For this review, take the finished solid that the model builds, in its own axes (mm). Round coordinates to 2 decimals unless told otherwise and drop trailing zeros. Order: outer loops, then holes, each group sorted by start corner. A loop starts at its lowest first (then second) coordinate and runs counter-clockwise, first axis right, second up. Notation, with made-up numbers: (-29.75, 57.25) -> (17.25, 57.25) arc R26 ccw to (17.25, 80.25) -> close; hole circle Ø5 at (-20, 45). An arc over 180 degrees is marked (long way). Answer in a Markdown table with one row per item.
```python
from build123d import *

# Parameters (mm, degrees)
SKETCH1_R               = 2
BOSS_EXTRUDE1_DEPTH     = 4
BOSS_EXTRUDE2_DEPTH     = 6
CUT_EXTRUDE1_START      = -2
CUT_EXTRUDE1_DEPTH      = 18
SKETCH4_W               = 12.2
SKETCH4_H               = 11
CUT_EXTRUDE2_DEPTH      = 10
SKETCH5_W               = 20
SKETCH5_H               = 2
BOSS_EXTRUDE3_DEPTH     = 35
CUT_EXTRUDE4_START      = -0.7
CUT_EXTRUDE4_DEPTH      = 0.7
CUT_EXTRUDE5_DEPTH      = 1
CUT_EXTRUDE6_REACH      = 144.046
SKETCH12_W              = 87
SKETCH12_H              = 2
FILLET1_R               = 10
CUT_EXTRUDE7_DEPTH      = 112.736296699
SKETCH14_W              = 20
SKETCH14_H              = 2
CUT_EXTRUDE8_DEPTH      = 142.58036587
FILLET2_R               = 10
CUT_EXTRUDE9_DEPTH      = 142.58036587
CUT_EXTRUDE9_DEPTH_BACK = 142.58036587
SKETCH15_W              = 20
SKETCH15_H              = 8
CUT_EXTRUDE10_REACH     = 143.58
SKETCH16_W              = 20
SKETCH16_H              = 2


with BuildPart() as part:
    # Sketch1 → Boss-Extrude1 (new, symmetric)
    with BuildSketch(Plane(origin=(0, 0, 0), x_dir=(1, 0, 0), z_dir=(0, 1, 0))):
        with BuildLine():
            ThreePointArc((-4, 7.5), (-11.5, 0), (-4, -7.5))
            Line((-4, -7.5), (0, -7.5))
            Line((0, -7.5), (0, 7.5))
            Line((0, 7.5), (-4, 7.5))
        make_face()
        with Locations(Location((-4, 0, 0), (0, 0, 270))):
            Circle(SKETCH1_R, mode=Mode.SUBTRACT)
    extrude(amount=BOSS_EXTRUDE1_DEPTH, both=True)

    # Sketch1<3> → Boss-Extrude2 (add, symmetric)
    with BuildSketch(Plane(origin=(0, 0, 0), x_dir=(1, 0, 0), z_dir=(0, 1, 0))):
        Polygon((0, 10), (0, 7.5), (0, 0), (141, 0), (141, 10), align=None)
        Polygon((0, 0), (0, -7.5), (0, -10), (141, -10), (141, 0), align=None)
    extrude(amount=BOSS_EXTRUDE2_DEPTH, both=True)

    # Sketch3 → Cut-Extrude1 (cut)
    with BuildSketch(Plane.ZY.offset(CUT_EXTRUDE1_START)):
        with BuildLine():
            Line((-3.494281042, -5), (3.494281042, -5))
            ThreePointArc((3.494281042, -5), (5.4094877, -2.819120931), (6.1, 0))
            Line((6.1, 0), (6.1, 6))
            Line((6.1, 6), (-6.1, 6))
            Line((-6.1, 6), (-6.1, 0))
            ThreePointArc((-6.1, 0), (-5.4094877, -2.819120931), (-3.494281042, -5))
        make_face()
    extrude(amount=-CUT_EXTRUDE1_DEPTH, mode=Mode.SUBTRACT)

    # Sketch4 → Cut-Extrude2 (cut)
    with BuildSketch(Plane.ZY.offset(-20)):
        with Locations((0, 0.5)):
            Rectangle(SKETCH4_W, SKETCH4_H)
    extrude(amount=-CUT_EXTRUDE2_DEPTH, mode=Mode.SUBTRACT)

    # Sketch5 → Boss-Extrude3 (add)
    with BuildSketch(Plane.ZY):
        with Locations((0, -7)):
            Rectangle(SKETCH5_W, SKETCH5_H)
    extrude(amount=-BOSS_EXTRUDE3_DEPTH)

    # Sketch9 → Cut-Extrude4 (cut)
    with BuildSketch(Plane(origin=(2, 0, 0), x_dir=(0, 0, -1), z_dir=(1, 0, 0)).offset(CUT_EXTRUDE4_START)):
        with BuildLine():
            Line((3.494281042, -5), (-3.494281042, -5))
            ThreePointArc((-3.494281042, -5), (-6.1, 0), (-3.494281042, 5))
            Line((-3.494281042, 5), (3.494281042, 5))
            ThreePointArc((3.494281042, 5), (6.1, 0), (3.494281042, -5))
        make_face()
    extrude(amount=CUT_EXTRUDE4_DEPTH, mode=Mode.SUBTRACT)

    # Sketch11 → Cut-Extrude5 (cut, symmetric)
    with BuildSketch(Plane(origin=(0, 0, 0), x_dir=(1, 0, 0), z_dir=(0, 1, 0))):
        with BuildLine():
            Line((2, 1), (2, -1))
            ThreePointArc((2, -1), (0.585786391, -1.585786484), (0, -3.000000131))
            Line((0, -3.000000131), (0, -7.5))
            Line((0, -7.5), (-2, -7.5))
            Line((-2, -7.5), (-2, -3.000000131))
            ThreePointArc((-2, -3.000000131), (-0.828427171, -0.171572922), (2, 1))
        make_face()
    extrude(amount=CUT_EXTRUDE5_DEPTH, both=True, mode=Mode.SUBTRACT)

    # Sketch12 → Cut-Extrude6 (cut, up to next)
    with BuildSketch(Plane(origin=(0, 6, 0), x_dir=(1, 0, 0), z_dir=(0, 1, 0)), mode=Mode.PRIVATE) as cut_extrude6_sk1:
        with Locations((97.5, 9)):
            Rectangle(SKETCH12_W, SKETCH12_H)
    cut_extrude6_tool1 = extrude(cut_extrude6_sk1.sketch, amount=-CUT_EXTRUDE6_REACH, mode=Mode.PRIVATE) & part.part
    # Sketch12 → Cut-Extrude6 (cut, up to next)
    with BuildSketch(Plane(origin=(0, 6, 0), x_dir=(1, 0, 0), z_dir=(0, 1, 0)), mode=Mode.PRIVATE) as cut_extrude6_sk2:
        with Locations((97.5, -9)):
            Rectangle(SKETCH12_W, SKETCH12_H)
    cut_extrude6_tool2 = extrude(cut_extrude6_sk2.sketch, amount=-CUT_EXTRUDE6_REACH, mode=Mode.PRIVATE) & part.part
    add(cut_extrude6_tool1.solids().sort_by_distance((97.5, 6, -9))[0], mode=Mode.SUBTRACT)
    add(cut_extrude6_tool2.solids().sort_by_distance((97.5, 6, 9))[0], mode=Mode.SUBTRACT)

    # Fillet1
    # the kernel refuses this fillet: 10 mm, written as the material it adds along each edge
    with BuildSketch(Plane(origin=(54, 6, 8), x_dir=(0, 0, 1), z_dir=(0, -1, 0))) as fillet1_piece_1:
        with BuildLine():
            CenterArc((10, -6), FILLET1_R, 143.130102354, 36.869897646)
            Line((0, -6), (-0.2, -6))
            Line((-0.2, -6), (-0.2, 0))
            Line((-0.2, 0), (0, 0.2))
            ThreePointArc((0, 0.2), (1, 0.2), (1.84, 0.12))
            Line((1.84, 0.12), (2, 0))
        make_face()
    extrude(amount=12)
    with BuildSketch(Plane(origin=(54, 6, -8), x_dir=(0, 0, -1), z_dir=(0, -1, 0))) as fillet1_piece_2:
        with BuildLine():
            CenterArc((10, 6), FILLET1_R, 180, 36.869897646)
            Line((0, 6), (-0.2, 6))
            Line((-0.2, 6), (-0.2, 0))
            Line((-0.2, 0), (0, -0.2))
            ThreePointArc((0, -0.2), (1, -0.2), (1.84, -0.12))
            Line((1.84, -0.12), (2, 0))
        make_face()
    extrude(amount=12)

    # Sketch13 → Cut-Extrude7 (cut, through all)
    with BuildSketch(Plane.ZY.offset(-30)):
        Polygon((-5, 5), (-5, 1), (-3.5, 1), (-3.5, -1), (-5, -1), (-5, -5), (5, -5), (5, -1), (3.5, -1), (3.5, 1), (5, 1), (5, 5), align=None)
    extrude(amount=-CUT_EXTRUDE7_DEPTH, mode=Mode.SUBTRACT)

    # Sketch14 → Cut-Extrude8 (cut, through all)
    with BuildSketch(Plane.ZY):
        with Locations((0, 5)):
            Rectangle(SKETCH14_W, SKETCH14_H)
    extrude(amount=-CUT_EXTRUDE8_DEPTH, mode=Mode.SUBTRACT)

    # Fillet2
    # the kernel refuses this fillet: 10 mm, written as the material it adds along each edge
    with BuildSketch(Plane(origin=(35, -6, -10), x_dir=(1, 0, 0), z_dir=(0, 0, 1))) as fillet2_piece_1:
        with BuildLine():
            CenterArc((6, -10), FILLET2_R, 90, 36.869897646)
            Line((0, -2), (-0.12, -1.84))
            ThreePointArc((-0.12, -1.84), (-0.2, -1), (-0.2, 0))
            Line((-0.2, 0), (0, 0.2))
            Line((0, 0.2), (6, 0.2))
            Line((6, 0.2), (6, 0))
        make_face()
    extrude(amount=20)

    # Sketch15 → Cut-Extrude9 (cut, two sides: drawn at the far end of the back side and taken through both)
    with BuildSketch(Plane(origin=(0, 0, 0), x_dir=(0, 0, -1), z_dir=(1, 0, 0)).offset(-CUT_EXTRUDE9_DEPTH_BACK)):
        Rectangle(SKETCH15_W, SKETCH15_H)
    extrude(amount=CUT_EXTRUDE9_DEPTH + CUT_EXTRUDE9_DEPTH_BACK, mode=Mode.SUBTRACT)

    # Sketch16 → Cut-Extrude10 (cut, up to next)
    with BuildSketch(Plane(origin=(0, 0, 0), x_dir=(0, 0, -1), z_dir=(1, 0, 0)), mode=Mode.PRIVATE) as cut_extrude10_sk1:
        with Locations((0, -7)):
            Rectangle(SKETCH16_W, SKETCH16_H)
    cut_extrude10_tool1 = extrude(cut_extrude10_sk1.sketch, amount=CUT_EXTRUDE10_REACH, mode=Mode.PRIVATE) & part.part
    add(cut_extrude10_tool1.solids().sort_by_distance((0, -7, 0))[0], mode=Mode.SUBTRACT)


solid = part.part
```
Q1. Take a section at B-B, the plane z = 0.25. Write out the cut boundary in (x, y).
Answer key:
| item | result |
|---|---|
| outline | (0, -6) -> (141, -6) -> (141, -5) -> (1.3, -5) -> (1.3, -4) -> (0, -4) -> close |
Q2. Clearance check with flat-ended pins moving along their axes: pin 1 Ø0.6 at (x, y) = (88, -5) entering from -Z; pin 2 Ø0.8 at (y, z) = (-4.5, 4.5) entering from +X; pin 3 Ø6 at (x, z) = (90, -0.5) entering from +Y. State where each tip first meets the part, or that it passes through.
Answer key:
| item | result |
|---|---|
| pin 1 | stops at z = -8 |
| pin 2 | stops at x = 20 |
| pin 3 | stops at y = -5 |
Q3. To check wall thickness, follow probe 1 along X at (y, z) = (-4.05, -6); probe 2 along Z at (x, y) = (31, -4.85); probe 3 along Z at (x, y) = (21.5, -4.8). State the ranges of each line that lie inside material, in increasing order.
Answer key:
| item | result |
|---|---|
| probe 1 | x = 0 to 20, 30 to 141 |
| probe 2 | z = -10 to -5, 5 to 10 |
| probe 3 | z = -10 to -6.1, 6.1 to 10 |
Q4. The part is to be moulded in two halves that separate along Z. For faces 1 (the face through (70, -5, 0)), 2 (the face through (71, -6, 0)), say which applies: +Z half, -Z half, draft (parallel to the pull), parting line (faces both ways), or undercut.
Answer key:
| item | result |
|---|---|
| face 1 | undercut |
| face 2 | draft |
Q5. Take a section at C-C, the plane y = -5.6. Write out the cut boundary in (x, z).
Answer key:
| item | result |
|---|---|
| outline | (0, -10) -> (54, -10) arc R10 cw to (60, -8) -> (141, -8) -> (141, 8) -> (60, 8) arc R10 cw to (54, 10) -> (0, 10) -> close |
Q6. Take a section at A-A, the plane x = 77. Write out the cut boundary in (y, z), then the cut area to 3 significant figures.
Answer key:
| item | result |
|---|---|
| outline | (-6, -8) -> (-4, -8) -> (-4, -5) -> (-5, -5) -> (-5, 5) -> (-4, 5) -> (-4, 8) -> (-6, 8) -> close |
| area | 22.0 mm^2 |
